Geometry: final body of the model. Coordinates: model frame, mm. Coordinates: 2 decimals unless noted, no trailing zeros. Write each loop counter-clockwise with the first axis right and the second up, starting at its lowest first coordinate (ties: lowest second). Pieces come first, ordered by that corner, then holes. Notation, with made-up numbers: (-31.75, -2) - (21.25, -2) arc R6 cw to (21.25, 8) - close; hole circle Ø7 at (-15, 70). An arc over 180 degrees is marked (long way). Answer as a JSON object with one key per item and string values. Group by question number.
Item 1: Line query: line 1 along X through (y, z) = (-12, 0.4); line 2 along Y through (x, z) = (8.5, 0.35); line 3 along Y through (x, z) = (8.25, 1.45). Output: solid intervals per line, ascending. Write a range as from..to.
Item 2: Section A-A on y = -12.25. Return loops of the section in (x, z).
Item 3: First-contact query: pin 1 Ø0.7 at (x, z) = (19, 1) entering from +Y. Flat tip, straight axial feed; report the tip coordinate or a pass-through.
Item 4: Section D-D on z = 0.25. State how many separate pieces and enclosed holes the cut face has, and give its area (3 significant figures).
Item 5: Section B-B on x = 19.25. Return loops of the section in (y, z).
Item 6: Section C-C on y = -7. Return loops of the section in (x, z), and give its area (3 significant figures).
```python
from build123d import *

# Parameters (mm, degrees)
F0_R     = 1.5875
F1_DEPTH = 1.524
F3_R     = 1.0471954036
F4_DEPTH = 1.525
F7_DEPTH = 1.524


with BuildPart() as f1:
    # F0 (on Top) → F1 (new body)
    with BuildSketch(Plane.XY):
        Polygon((12.3030065617, -0.1368533121), (2.0698180888, -0.1368533121), (2.0698180888, -18.6402630061), (6.0960869305, -18.6402630061), (6.0960869305, -15.829924494), (4.6535655856, -15.829924494), (4.6535655856, -14.3967131153), (6.0960869305, -14.3967131153), (6.0960869305, -11.3862287253), (9.2548192479, -11.3862287253), (9.2548192479, -18.5830555856), (12.3030065617, -18.5830555856), align=None)
        with Locations((4.1468967684, -2.2560383659)):
            Circle(F0_R, mode=Mode.SUBTRACT)
    extrude(amount=F1_DEPTH)

    # F2: F1 across face


with BuildPart() as f1_1:
    add(f1.part)
    add(f1.part.mirror(Plane(origin=(12.3030065617, -9.3599544489, 0.762), x_dir=(0, 1, 0), z_dir=(1, 0, 0))))

    # F3 (on face) → F4 (cut, through all)
    with BuildSketch(Plane(origin=(0, 0, 0), x_dir=(1, 0, 0), z_dir=(0, 0, -1))):
        with Locations((16.1656420678, 3.8247841876)):
            Circle(F3_R)
        with BuildLine():
            ThreePointArc((13.5849428674, 4.8719795912), (12.8444638963, 3.0843052165), (14.6321382709, 3.8247841876))
            ThreePointArc((14.6321382709, 3.8247841876), (14.3254218385, 4.5652631587), (13.5849428674, 4.8719795912))
        make_face()
        with BuildLine():
            ThreePointArc((14.6321382709, 6.3911853358), (12.8444638963, 7.1316643069), (13.5849428674, 5.3439899322))
            ThreePointArc((13.5849428674, 5.3439899322), (14.3254218385, 5.6507063647), (14.6321382709, 6.3911853358))
        make_face()
        with Locations((8.4235444665, 3.8247841876)):
            Circle(F3_R)
        with Locations((8.4235444665, 6.3911853358)):
            Circle(F3_R)
        with Locations((16.1656420678, 6.3911853358)):
            Circle(F3_R)
        with BuildLine():
            ThreePointArc((11.0042436669, 4.8719795912), (10.2637646958, 3.0843052165), (12.0514390705, 3.8247841876))
            ThreePointArc((12.0514390705, 3.8247841876), (11.744722638, 4.5652631587), (11.0042436669, 4.8719795912))
        make_face()
        with BuildLine():
            ThreePointArc((12.0514390705, 6.3911853358), (10.2637646958, 7.1316643069), (11.0042436669, 5.3439899322))
            ThreePointArc((11.0042436669, 5.3439899322), (11.744722638, 5.6507063647), (12.0514390705, 6.3911853358))
        make_face()
    extrude(amount=-F4_DEPTH, mode=Mode.SUBTRACT)

    # F6 (on face) → F7 (join, through all)
    with BuildSketch(Plane.XY.offset(1.524)):
        Polygon((2.7463897519, 1.0350031834), (2.0698180888, -0.1368533121), (2.949699899, -0.1368533121), (3.4063011096, 0.6540031834), align=None)
    extrude(amount=-F7_DEPTH)


solid = f1_1.part
```
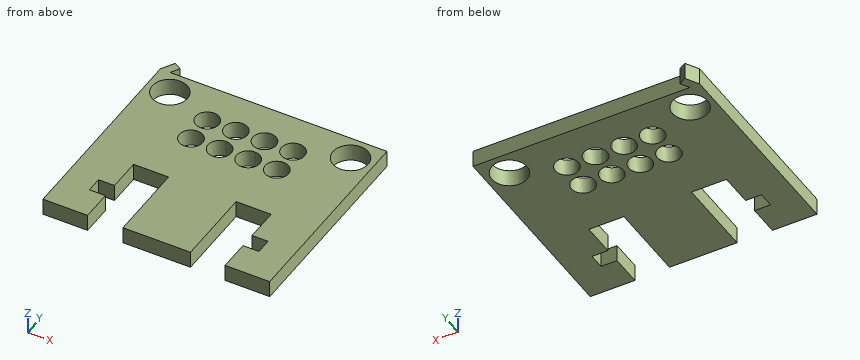
Checks:
{
 "1": {"line 1": "2.07..6.1, 9.25..15.35, 18.51..22.54", "line 2": "-11.39..-7.44, -5.35..-4.87, -2.78..-0.14", "line 3": "-11.39..-7.42, -5.36..-4.86, -2.79..-0.14"},
 "2": {"outline": "(2.07, 0) - (6.1, 0) - (6.1, 1.52) - (2.07, 1.52) - close; (9.25, 0) - (15.35, 0) - (15.35, 1.52) - (9.25, 1.52) - close; (18.51, 0) - (22.54, 0) - (22.54, 1.52) - (18.51, 1.52) - close"},
 "3": {"pin 1": "y = -0.14"},
 "4": {"separate pieces": "1", "enclosed holes": "10", "area": "286 mm^2"},
 "5": {"outline": "(-18.64, 0) - (-15.83, 0) - (-15.83, 1.52) - (-18.64, 1.52) - close; (-14.4, 0) - (-3.28, 0) - (-3.28, 1.52) - (-14.4, 1.52) - close; (-1.23, 0) - (-0.14, 0) - (-0.14, 1.52) - (-1.23, 1.52) - close"},
 "6": {"outline": "(2.07, 0) - (7.57, 0) - (7.57, 1.52) - (2.07, 1.52) - close; (9.28, 0) - (10.15, 0) - (10.15, 1.52) - (9.28, 1.52) - close; (11.86, 0) - (12.73, 0) - (12.73, 1.52) - (11.86, 1.52) - close; (14.44, 0) - (15.31, 0) - (15.31, 1.52) - (14.44, 1.52) - close; (17.02, 0) - (22.54, 0) - (22.54, 1.52) - (17.02, 1.52) - close", "area": "20.8 mm^2"}
}
